For this review, take the finished solid that the model builds, in its own axes (mm). A direction names the side the tool comes from. Give positions to 0.01 mm unless a question says otherwise; leave off trailing zeros. Loops run counter-clockwise (first coordinate to the right, second up) from the corner with the lowest first, then second, coordinate; pieces in that order, holes last.
```python
from build123d import *

# Parameters (mm, degrees)
F0_W     = 9.398
F0_H     = 19.05
F0_H_2   = 12.7
F0_W_2   = 9.652
F3_DEPTH = 25.4
F5_DEPTH = 12.7


with BuildPart() as f1:
    # F0 (on Front) → F1 (revolve)
    with BuildSketch(Plane.XZ):
        with Locations((-4.699, 9.525)):
            Rectangle(F0_W, F0_H)
        with Locations((-4.699, 25.4)):
            Rectangle(F0_W, F0_H_2)
        with Locations((-14.224, 9.525)):
            Rectangle(F0_W_2, F0_H)
        Polygon((-9.398, 31.75), (0, 31.75), (0, 50.8), (-9.398, 50.8), (-9.398, 44.45), (-12.446, 44.45), (-12.446, 38.1), (-9.398, 38.1), align=None)
        Polygon((-19.05, 19.05), (-9.398, 19.05), (-9.398, 31.75), (-19.05, 31.75), (-38.1, 31.75), (-38.1, 19.05), align=None)
        Polygon((-19.05, 31.75), (-9.398, 31.75), (-9.398, 38.1), (-12.446, 38.1), (-12.446, 44.45), (-9.398, 44.45), (-9.398, 50.8), (-19.05, 50.8), align=None)
    revolve(axis=Axis((0, 0, 25.4), (0, 0, 1)))

    # F2 (on face) → F3 (cut)
    with BuildSketch(Plane.XY.offset(31.75)):
        with BuildLine():
            Line((3.68e-08, 19.05), (32.9955678842, 19.05))
            ThreePointArc((32.9955678842, 19.05), (0, 38.1), (-32.9955678842, 19.05))
            Line((-32.9955678842, 19.05), (3.68e-08, 19.05))
        make_face()
        with BuildLine():
            ThreePointArc((-32.9955678842, -19.05), (0, -38.1), (32.9955678842, -19.05))
            Line((32.9955678842, -19.05), (3.68e-08, -19.05))
            Line((3.68e-08, -19.05), (-32.9955678842, -19.05))
        make_face()
    extrude(amount=-F3_DEPTH, mode=Mode.SUBTRACT)

    # F4 (on face) → F5 (join, through all)
    with BuildSketch(Plane.XY.offset(31.75)):
        with BuildLine():
            Line((-38.1, 19.05), (-38.1, 0))
            ThreePointArc((-38.1, 0), (-36.8017739816, 9.8610056184), (-32.9955678842, 19.05))
            Line((-32.9955678842, 19.05), (-38.1, 19.05))
        make_face()
        with BuildLine():
            ThreePointArc((-32.9955678842, -19.05), (-36.8017739816, -9.8610056184), (-38.1, 0))
            Line((-38.1, 0), (-38.1, -19.05))
            Line((-38.1, -19.05), (-32.9955678842, -19.05))
        make_face()
        with BuildLine():
            ThreePointArc((32.9955678842, 19.05), (36.8017739816, 9.8610056184), (38.1, 0))
            Line((38.1, 0), (38.1, 19.05))
            Line((38.1, 19.05), (32.9955678842, 19.05))
        make_face()
        with BuildLine():
            Line((38.1, -19.05), (38.1, 0))
            ThreePointArc((38.1, 0), (36.8017739816, -9.8610056184), (32.9955678842, -19.05))
            Line((32.9955678842, -19.05), (38.1, -19.05))
        make_face()
    extrude(amount=-F5_DEPTH)

    # F6 (on Front) → F7 (revolve, cut)
    with BuildSketch(Plane.XZ):
        Polygon((0, 50.8), (-9.398, 50.8), (-9.398, 44.45), (-12.446, 44.45), (-12.446, 38.1), (-9.398, 38.1), (-9.398, 0), (0, 0), align=None)
    revolve(axis=Axis((0, 0, 25.4), (0, 0, 1)), mode=Mode.SUBTRACT)


solid = f1.part
```
Item 1: The part is to be moulded in two halves that separate along X. For faces 1 (the flat face through (-38.1, 0, 25)), 2 (the cylindrical face through (1.22, -9.32, 47.58)), 3 (the flat face through (-4.6, -8.4, 38.1)), 4 (the flat face through (-28, 0, 31.75)), say which applies: released by +X, released by -X, zero draft, split by the parting line, or undercut.
Answer:
face 1: released by -X
face 2: undercut
face 3: undercut
face 4: zero draft
Item 2: Clearance check with flat-ended pins moving along their axes: pin 1 Ø4 at (x, z) = (-5.5, 15) entering from -Y; pin 2 Ø4 at (x, y) = (-23, 9) entering from -Z; pin 3 Ø2 at (y, z) = (12, 42.5) entering from -X. State where each tip first meets the part, or that it passes through.
Answer:
pin 1: stops at y = -18.73
pin 2: stops at z = 19.05
pin 3: stops at x = -15.55
Item 3: Take a section at A-A on y = 0. Give the boundary of the cut face in (x, z), and give its area (3 significant figures).
Answer:
outline: (-38.1, 19.05) - (-19.05, 19.05) - (-19.05, 0) - (-9.4, 0) - (-9.4, 38.1) - (-12.45, 38.1) - (-12.45, 44.45) - (-9.4, 44.45) - (-9.4, 50.8) - (-19.05, 50.8) - (-19.05, 31.75) - (-38.1, 31.75) - close; (9.4, 0) - (19.05, 0) - (19.05, 19.05) - (38.1, 19.05) - (38.1, 31.75) - (19.05, 31.75) - (19.05, 50.8) - (9.4, 50.8) - (9.4, 44.45) - (12.45, 44.45) - (12.45, 38.1) - (9.4, 38.1) - close
area: 1,430 mm2
Item 4: Tool access review of faces 5 (the flat face through (27, 0, 31.75)), 6 (the cylindrical face through (15.12, 11.59, 9.66)), 7 (the flat face through (4.6, -8.4, 44.45)), 8 (the cylindrical face through (15.12, 11.59, 41.14)), 9 (the flat face through (4, -9, 50.8)): name each direction out of +Z, -Z, +X, -X, +Y, -Y from which nothing blocks a thin tool from reaching the whole face with its end or side.
Answer:
face 5: +Z, +X
face 6: -Z
face 7: none
face 8: +Z
face 9: +Z, +X, -X, +Y, -Y
Item 5: For L1, parallel to Y at x = 0, z = 15; L2, parallel to X at y = 0, z = 43, list the stretches that pass through material, from the lowest coordinate up.
Answer:
L1: y = -19.05 to -9.4, 9.4 to 19.05
L2: x = -19.05 to -12.45, 12.45 to 19.05
Item 6: Take a section at B-B on x = -3. Give the boundary of the cut face in (y, z), and give its area (3 significant figures).
Answer:
outline: (-19.05, 19.05) - (-18.81, 19.05) - (-18.81, 0) - (-8.91, 0) - (-8.91, 38.1) - (-12.08, 38.1) - (-12.08, 44.45) - (-8.91, 44.45) - (-8.91, 50.8) - (-18.81, 50.8) - (-18.81, 31.75) - (-19.05, 31.75) - close; (8.91, 0) - (18.81, 0) - (18.81, 19.05) - (19.05, 19.05) - (19.05, 31.75) - (18.81, 31.75) - (18.81, 50.8) - (8.91, 50.8) - (8.91, 44.45) - (12.08, 44.45) - (12.08, 38.1) - (8.91, 38.1) - close
area: 972 mm2
Item 7: Take a section at C-C on z = 28.5. Give the boundary of the cut face in (x, y).
Answer:
outline: (-38.1, -19.05) - (38.1, -19.05) - (38.1, 19.05) - (-38.1, 19.05) - close; hole circle Ø18.8 at (0, 0)
Item 8: Take a section at D-D on y = -11.5. Give the boundary of the cut face in (x, z), and give its area (3 significant figures).
Answer:
outline: (-38.1, 19.05) - (-15.19, 19.05) - (-15.19, 0) - (15.19, 0) - (15.19, 19.05) - (38.1, 19.05) - (38.1, 31.75) - (15.19, 31.75) - (15.19, 50.8) - (-15.19, 50.8) - (-15.19, 31.75) - (-38.1, 31.75) - close; hole (-4.76, 38.1) - (4.76, 38.1) - (4.76, 44.45) - (-4.76, 44.45) - close
area: 2,060 mm2
